Autodesk Inventor part; units mm, degrees
ref_plane "YZ Plane" through (0, 0, 0) normal (1, 0, 0) x (0, 1, 0)
ref_plane "XZ Plane" through (0, 0, 0) normal (0, 1, 0) x (-1, 0, 0)
ref_plane "XY Plane" through (0, 0, 0) normal (0, 0, 1) x (1, 0, 0)
ref_plane "Work Plane1" through (400, -8.5282, -0.75) normal (1, 0, 0) x (0, 0.7071068, -0.7071068)
sketch "Sketch1" plane through (400, -8.5282, -0.75) normal (1, 0, 0) x (0, 0.7071068, -0.7071068)
  line L0 (-10.9826, 10.0209) -> (10.0174, 10.0209)
  line L1 (10.0174, 10.0209) -> (10.0174, -9.9791)
  line L2 (10.0174, -9.9791) -> (-10.9826, -9.9791)
  line L3 (-10.9826, -9.9791) -> (-10.9826, 10.0209)
  line L4 (10.0174, 10.0209) -> (13.0174, 10.0209)
  line L5 (13.0174, 10.0209) -> (13.0174, -9.9791)
  line L6 (13.0174, -9.9791) -> (10.0174, -9.9791)
  line L7 (10.0174, -9.9791) -> (10.0174, 10.0209)
  line L8 (-10.9826, 10.0209) -> (-13.9826, 10.0209)
  line L9 (-13.9826, 10.0209) -> (-13.9826, -9.9791)
  line L10 (-13.9826, -9.9791) -> (-10.9826, -9.9791)
  line L11 (-10.9826, -9.9791) -> (-10.9826, 10.0209)
  point P0 (5.5, 6.5607)
  point P1 (10.0174, -9.9791)
  point P2 (-10.9826, -9.9791)
  dimension "d0" = 21
  dimension "d1" = 20
  dimension "d2" = 3
  dimension "d3" = 20
  dimension "d4" = 3
  dimension "d5" = 20
extrude "Extrusion1" add sketch "Sketch1" against normal blind 30 contours L3 L10 L9 L8 | L4 L5 L6 L1
sketch "Sketch2" plane through (400, -8.5282, -0.75) normal (1, 0, 0) x (0, -0.7071068, -0.7071068)
  line L0 (-10.0209, -13.9826) -> (-10.0209, -10.9826)
  line L1 (9.9791, 13.0174) -> (9.9791, 10.0174)
  line L2 (-10.0209, -13.9826) -> (9.9791, -13.9826)
  line L3 (9.9791, -13.9826) -> (9.9791, 13.0174)
  line L4 (9.9791, 13.0174) -> (-10.0209, 13.0174)
  line L5 (-10.0209, 13.0174) -> (-10.0209, -13.9826)
  point P0 (-6.5607, 5.5)
extrude "Extrusion2" add sketch "Sketch2" along normal blind 5
sketch "Sketch3" plane through (405, -6.3798, -17.011) normal (0, -0.7071068, -0.7071068) x (-1, 0, 0)
  line L0 (35, 0) -> (0, 0)
  line L1 (0, 0) -> (-15, 0)
  line L2 (-15, 0) -> (-15, -26)
  line L3 (-15, -26) -> (0, -26)
  line L4 (0, -26) -> (0, 0)
  line L5 (-10.0102, -5) -> (0, -5)
  line L6 (0, -5) -> (0, -21)
  line L7 (0, -21) -> (-10.0102, -21)
  line L8 (-10.0102, -21) -> (-10.0102, -5)
  point P0 (405, -7.5174)
  point P1 (0, -21)
  point P2 (0, -5)
  dimension "d10" = 15
  dimension "d11" = 26
  dimension "d12" = 0
  dimension "d13" = 5
  dimension "d14" = 16
extrude "Extrusion3" add sketch "Sketch3" against normal blind 8 contours L4 L5 L8 L7 L3 L2 L1
sketch "Sketch4" plane through (370, -11.3295, 16.223) normal (0, -0.7071068, 0.7071068) x (1, 0, 0)
  circle A0 centre (15, -10) radius 2.75
  line L0 (0, -20) -> (50, -20)
  line L1 (0, -20) -> (0, 0)
  point P0 (-370, -3.4602)
  dimension "d17" = 5.5
  dimension "d18" = 10
  dimension "d19" = 15
extrude "Extrusion4" cut sketch "Sketch4" against normal through all
sketch "Sketch5" plane through (370, -11.3295, 16.223) normal (0, -0.7071068, 0.7071068) x (1, 0, 0)
  circle A0 centre (15, -10) radius 2.75
  circle A1 centre (15, -10) radius 5.75
  point P0 (-370, -3.4602)
  dimension "d22" = 11.5
extrude "Extrusion5" cut sketch "Sketch5" against normal blind 1 contours A0 | A1
sketch "Sketch6" plane through (405, 7.7624, -2.8688) normal (0, 0.7071068, -0.7071068) x (-1, 0, 0)
  circle A0 centre (20, -10) radius 2.75
  circle A1 centre (20, -10) radius 5.75
  point P0 (405, -3.4602)
  dimension "d25" = 11.5
extrude "Extrusion6" cut sketch "Sketch6" against normal blind 1
equation "\"d14\" = d11 - 2 * d13"
properties part number "StrapHolder"
Part model, mm, in its own coordinate system. A direction names the side the tool comes from. Coordinates: 2 decimals unless noted, no trailing zeros. Order: outer loops, then holes, each group sorted by start corner. A loop starts at its lowest first (then second) coordinate and runs counter-clockwise, first axis right, second up. Notation, with made-up numbers: M 4.25,-34 L 28.25,-34 A25 cw 28.25,-18 Z; hole C -12,34 d6. An arc over 180 degrees is marked long. Use a Markdown table: item, result.
(1) Pull direction X, two halves, no side cores. Call faces 6 (the flat face through (388.54, -16.38, 6.93)), 7 (the flat face through (382.364, -16.732, 9.404)), 8 (the flat face through (370, -17, 8)), 9 (the flat face through (409.94, -18.44, 0.63)): released by +X, released by -X, zero draft, split by the parting line, or undercut.
A:
| item | result |
|---|---|
| face 6 | zero draft |
| face 7 | undercut |
| face 8 | released by -X |
| face 9 | undercut |
(2) Flat gauge pins, fed straight in: pin 1 (9 mm diameter, centred on y = -5.5, z = 0.5, fed in from +X); pin 2 (3 mm diameter, centred on x = 414.5, y = -21.5, fed in from +Z); pin 3 (5 mm diameter, centred on x = 385.5, y = -18.5, fed in from -Z). Where does each tip first touch, or does it go through?
A:
| item | result |
|---|---|
| pin 1 | stops at x = 405 |
| pin 2 | stops at z = 6.14 |
| pin 3 | stops at z = 2.31 |
(3) Probe L1, parallel to X at y = -14, z = 4; L2, parallel to Y at x = 376, z = -12; L3, parallel to Y at x = 392, z = -5. List the from-to ranges inside material, lowest first.
A:
| item | result |
|---|---|
| L1 | x = 400 to 405 |
| L2 | y = -5.61 to -1.37 |
| L3 | y = 1.39 to 5.63 |
(4) Tool access for faces 1 (the flat face through (400, -9, 0)), 2 (the flat face through (387.636, 0.943, -8.271)), 3 (the flat face through (410.08, -7.13, -10.69)), 4 (the flat face through (388.54, -1.33, -7.72)), 5 (the flat face through (415.938, -9.787, -2.29)): list every direction of +Z, -Z, +X, -X, +Y, -Y with a clear straight run to the whole face (end or side of a thin tool).
A:
| item | result |
|---|---|
| face 1 | -X |
| face 2 | none |
| face 3 | +Z, -Y |
| face 4 | +Z, -X, -Y |
| face 5 | +Z, +X, +Y |
(5) Cut at A-A on x = 375.5. Write the cut outline in (y, z).
A:
| item | result |
|---|---|
| outline | M -25.47,2.08 L -23.35,-0.04 L -9.21,14.1 L -11.33,16.22 Z; M -8.5,-14.89 L -6.38,-17.01 L 7.76,-2.87 L 5.64,-0.75 Z |
